Read the model definition and answer for the solid it produces. Units are mm, in the model's axes. Face numbers are marked on the shaded views. A direction names the side the tool comes from. Give positions to 0.01 mm unless a question says otherwise; leave off trailing zeros. Loops run counter-clockwise (first coordinate to the right, second up) from the corner with the lowest first, then second, coordinate; pieces in that order, holes last.
(1) Find section C-C, the plane y = -4.5. Write down the section's boundary in (x, z), then the cut area to 3 significant figures.
(2) Straight lines are drawn through the part: probe 1 along Y at (x, z) = (0, 2.5); probe 2 along X at (y, z) = (8.5, 4); probe 3 along Y at (x, z) = (-8, 4). For each, find the intervals that lie inside material, in ascending order.
(3) Find section B-B, the plane z = 1.5. Write down the section's boundary in (x, y), then the cut area to 3 significant figures.
(4) Each of these flat-tipped pins is pushed along its axis until it touches: P1, Ø5, axis at x = -2.5, z = 7, coming from the +Y side; P2, Ø4.5, axis at x = -19, z = 6.5, coming from the +Y side; P3, Ø4, axis at y = 10, z = 7, coming from the -X side; P4, Ø3, axis at y = -2.5, z = 5, coming from the +X side. Where does it stop, or does it pass through?
(5) Determine the mould class of the marked faces 1, 2, 3 and 4 for opening direction X: pulls with the +X half, pulls with the -X half, needs draft (parallel to the pull), parting line crosses it, or undercut.
(6) Find section D-D, the plane x = 18.5. Write down the section's boundary in (y, z).
(7) Find section A-A, the plane x = 0. Write down the section's boundary in (y, z).
(8) Which of the six approach directions +Z, -Z, +X, -X, +Y, -Y give full straight-line access (tool end or side, diameter ignored) to the marked faces 5, 6 and 7?
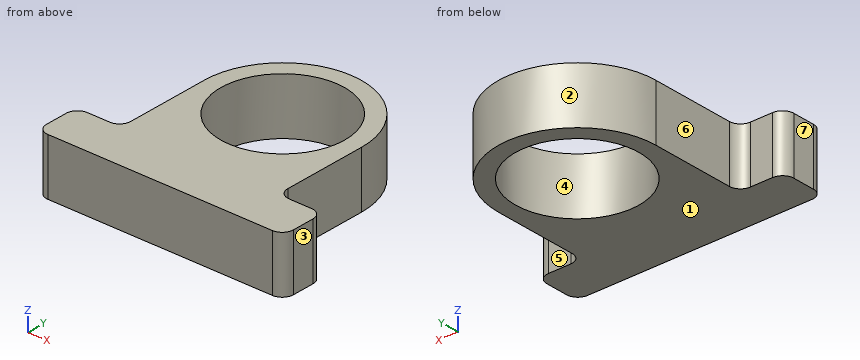
```python
from build123d import *

# Parameters (mm, degrees)
SKETCH1_R           = 14
SKETCH1_R_2         = 11
BOSS_EXTRUDE1_DEPTH = 10
FILLET1_R           = 2


with BuildPart() as part:
    # Sketch1 → Boss-Extrude1 (new body)
    # profile 1 of 2: a face of its own
    with BuildSketch(Plane.XY):
        with BuildLine():
            ThreePointArc((14, 0), (0, -14), (-14, 0))
            Line((-14, 0), (-14, -17))
            Line((-14, -17), (-22, -17))
            Line((-22, -17), (-22, -25))
            Line((-22, -25), (22, -25))
            Line((22, -25), (22, -17))
            Line((22, -17), (14, -17))
            Line((14, -17), (14, 0))
        make_face()
    # profile 2 of 2: a face of its own
    with BuildSketch(Plane.XY):
        Circle(SKETCH1_R)
        Circle(SKETCH1_R_2, mode=Mode.SUBTRACT)
    extrude(amount=BOSS_EXTRUDE1_DEPTH)

    # Fillet1
    fillet1_edges = [part.edges().sort_by_distance(p)[0] for p in [
        (14, -17, 5),
        (22, -17, 5),
        (22, -25, 5),
        (-22, -25, 5),
        (-22, -17, 5),
        (-14, -17, 5),
    ]]
    fillet(fillet1_edges, radius=FILLET1_R)


solid = part.part
```
Entries:
1. outline: (-14, 0) - (-10.04, 0) - (-10.04, 10) - (-14, 10) - close; (10.04, 0) - (14, 0) - (14, 10) - (10.04, 10) - close
1. area: 79.3 mm2
2. probe 1: y = -25 to -11, 11 to 14
2. probe 2: x = -11.12 to -6.98, 6.98 to 11.12
2. probe 3: y = -25 to -7.55, 7.55 to 11.49
3. outline: (-22, -23) arc R2 ccw to (-20, -25) - (20, -25) arc R2 ccw to (22, -23) - (22, -19) arc R2 ccw to (20, -17) - (16, -17) arc R2 cw to (14, -15) - (14, 0) arc R14 ccw to (-14, 0) - (-14, -15) arc R2 cw to (-16, -17) - (-20, -17) arc R2 ccw to (-22, -19) - close; hole circle Ø22 at (0, 0)
3. area: 754 mm2
4. P1: stops at y = 14
4. P2: stops at y = -17
4. P3: stops at x = -11.49
4. P4: stops at x = 14
5. face 1: needs draft
5. face 2: parting line crosses it
5. face 3: pulls with the +X half
5. face 4: undercut
6. outline: (-25, 0) - (-17, 0) - (-17, 10) - (-25, 10) - close
7. outline: (-25, 0) - (-11, 0) - (-11, 10) - (-25, 10) - close; (11, 0) - (14, 0) - (14, 10) - (11, 10) - close
8. face 5: +Z, -Z, +X, +Y
8. face 6: +Z, -Z, -X, +Y
8. face 7: +Z, -Z, -X, +Y, -Y
